from build123d import *

# Parameters (mm, degrees)
ESBO_O1_W                     = 13
ESBO_O1_H                     = 15
RESSALTO_EXTRUS_O1_DEPTH      = 9.5
ESBO_O3_R                     = 6.25
CORTE_EXTRUS_O1_DEPTH         = 10.5
ESBO_O2_W                     = 3
ESBO_O2_H                     = 4
ESBO_O2_R                     = 0.75
RESSALTO_EXTRUS_O2_DEPTH      = 8
RESSALTO_EXTRUS_O2_DEPTH_BACK = 9.5
RESSALTO_EXTRUS_O3_DEPTH      = 1.5
ESBO_O5_W                     = 12
ESBO_O5_H                     = 10
ESBO_O5_W_2                   = 10
ESBO_O5_H_2                   = 8
RESSALTO_EXTRUS_O4_DEPTH      = 7.5
RESSALTO_EXTRUS_O5_DEPTH      = 1
FILETE1_R                     = 1


with BuildPart() as part:
    # Esbo_o1 → Ressalto-extrus_o1 (new body)
    with BuildSketch(Plane.XY):
        Rectangle(ESBO_O1_W, ESBO_O1_H)
    extrude(amount=-RESSALTO_EXTRUS_O1_DEPTH)

    # Esbo_o3 → Corte-extrus_o1 (cut, through all)
    with BuildSketch(Plane.XY):
        Circle(ESBO_O3_R)
    extrude(amount=-CORTE_EXTRUS_O1_DEPTH, mode=Mode.SUBTRACT)

    # Esbo_o4 → Ressalto-extrus_o3 (add)
    with BuildSketch(Plane.ZY.offset(6.5)):
        Polygon((-6.5, 2.25), (-6.5, -1.75), (-4.849272887, -0.75), (-4.849272887, 1.25), align=None)
    extrude(amount=RESSALTO_EXTRUS_O3_DEPTH)

    # Esbo_o5 → Ressalto-extrus_o4 (add)
    with BuildSketch(Plane(origin=(0, 0, -9.5), x_dir=(-1, 0, 0), z_dir=(0, 0, -1))):
        Rectangle(ESBO_O5_W, ESBO_O5_H)
        Rectangle(ESBO_O5_W_2, ESBO_O5_H_2, mode=Mode.SUBTRACT)
    extrude(amount=-RESSALTO_EXTRUS_O4_DEPTH)



with BuildPart() as body_2:
    # Esbo_o2 → Ressalto-extrus_o2 (new body, two sides)
    with BuildSketch(Plane.XY) as ressalto_extrus_o2_sk:
        Rectangle(ESBO_O2_W, ESBO_O2_H)
        Circle(ESBO_O2_R, mode=Mode.SUBTRACT)
    extrude(amount=RESSALTO_EXTRUS_O2_DEPTH)
    extrude(ressalto_extrus_o2_sk.sketch, amount=-RESSALTO_EXTRUS_O2_DEPTH_BACK)


with BuildPart() as part_1:
    add(part.part)

    add(body_2.part)  # Ressalto-extrus_o5 merges body 2
    # Esbo_o6 → Ressalto-extrus_o5 (add)
    with BuildSketch(Plane.ZY.offset(1.5)):
        Polygon((-1, 7.5), (-1, 6.5), (2, 3.667217521), (2, -3.332782479), (-1, -6.5), (-1, -7.5), (-2, -7.5), (-2, -6.101577834), (1, -2.934360312), (1, 3.236113484), (-2, 6.068895963), (-2, 7.5), align=None)
    ressalto_extrus_o5 = extrude(amount=RESSALTO_EXTRUS_O5_DEPTH)

    # Espelhar1: Ressalto-extrus_o5 across plane
    add(ressalto_extrus_o5.mirror(Plane(origin=(0, 0, 0), x_dir=(0, 0, 1), z_dir=(1, 0, 0))))

    # Filete1
    filete1_edges = [part_1.edges().sort_by_distance(p)[0] for p in [
        (2, -3.332782479, 2),
        (2, 3.667217521, 2),
        (-2, -3.332782479, 2),
        (-2, 3.667217521, 2),
    ]]
    fillet(filete1_edges, radius=FILETE1_R)


solid = part_1.part
The listing builds one solid part. Answer for the finished solid, in the listing's coordinates (mm). A direction names the side the tool comes from. Round coordinates to 2 decimals unless told otherwise and drop trailing zeros. Write each loop counter-clockwise with the first axis right and the second up, starting at its lowest first coordinate (ties: lowest second). Pieces come first, ordered by that corner, then holes. Notation, with made-up numbers: (73.25, -2) - (77.25, -2) arc R31 ccw to (77.25, 22) - close; hole circle Ø2 at (-31, -39.75). An arc over 180 degrees is marked (long way). Use a Markdown table: item, result. Add a question column.
1. The part is cut by section D-D (z = 6.5). Write down the section's boundary in (x, y), and give its area (3 significant figures).
2. The part is cut by section A-A (x = 0). Write down the section's boundary in (y, z), and give its area (3 significant figures).
3. The part is cut by section C-C (y = -1.5). Give the number of separate pieces and of enclosed holes in the cut face, and give its area (3 significant figures).
4. Consider line 1 (Y direction, x = 0, z = -5); line 2 (Y direction, x = 1.75, z = -7); line 3 (X direction, y = 1, z = -5.5). Determine where each line is inside the solid, lowest interval first.
5. The part is cut by section B-B (z = -7). Write down the section's boundary in (x, y).
6. A tool of negligible diameter and unlimited length cuts with its end or side. For faces 4 (the face through (-1.5, 0, 5)), 5 (the face through (1.5, 0, -4)), 6 (the face through (5, 0, -6)), 7 (the face through (-1.993, 5.03, 0.557)), 8 (the face through (-1.99, -4.52, -0.5)), from which of +Z, -Z, +X, -X, +Y, -Y can it reach the whole face along a straight path? Write none if from no direction.
7. Flat-ended cylindrical pins translate along their axes: P1, Ø5, axis at x = -1, z = 3.5, coming from the +Y side; P2, Ø1, axis at y = -1, z = 4, coming from the -X side; P3, Ø0.8, axis at x = -5.5, y = -1.5, coming from the +Z side. Find the tip coordinate at first contact, or state that the pin passes through.
8. For a pull along Y with two mould halves and no side action, classify faces 1 (the face through (6.5, 0, -5)), 2 (the face through (-7.24, -1.26, -5.69)), 3 (the face through (0, 5, -6)) as +Y half, -Y half, draft (parallel to the pull), parting line (faces both ways), or undercut.
Reported:
| question | item | result |
|---|---|---|
| 1 | outline | (-1.5, -2) - (1.5, -2) - (1.5, 2) - (-1.5, 2) - close; hole circle Ø1.5 at (0, 0) |
| 1 | area | 10.2 mm^2 |
| 2 | outline | (-7.5, -9.5) - (-6.25, -9.5) - (-6.25, 0) - (-7.5, 0) - close; (-5, -9.5) - (-4, -9.5) - (-4, -2) - (-5, -2) - close; (-2, -9.5) - (-0.75, -9.5) - (-0.75, 8) - (-2, 8) - close; (0.75, -9.5) - (2, -9.5) - (2, 8) - (0.75, 8) - close; (4, -9.5) - (5, -9.5) - (5, -2) - (4, -2) - close; (6.25, -9.5) - (7.5, -9.5) - (7.5, 0) - (6.25, 0) - close |
| 2 | area | 82.5 mm^2 |
| 3 | separate pieces | 5 |
| 3 | enclosed holes | 0 |
| 3 | area | 78.3 mm^2 |
| 4 | line 1 | -7.5 to -6.25, -5 to -4, -2 to -0.75, 0.75 to 2, 4 to 5, 6.25 to 7.5 |
| 4 | line 2 | -7.5 to -6, -5 to -4, 4 to 5, 6 to 7.5 |
| 4 | line 3 | -8 to -6.17, -6 to -5, -1.5 to 1.5, 5 to 6, 6.17 to 6.5 |
| 5 | outline | (-6.5, -7.5) - (6.5, -7.5) - (6.5, 7.5) - (-6.5, 7.5) - close; (-1.5, -2) - (1.5, -2) - (1.5, 2) - (-1.5, 2) - close; hole (-6, -1.75) - (-6, 1.75) arc R6.25 ccw to start; hole (-5, -3.75) arc R6.25 ccw to (-4.8, -4) - (4.8, -4) arc R6.25 ccw to (5, -3.75) - (5, 3.75) arc R6.25 ccw to (4.8, 4) - (-4.8, 4) arc R6.25 ccw to (-5, 3.75) - close; hole (-3.75, -5) arc R6.25 ccw to (3.75, -5) - close; hole (-3.75, 5) - (3.75, 5) arc R6.25 ccw to start; hole circle Ø1.5 at (0, 0); hole (6, -1.75) arc R6.25 ccw to (6, 1.75) - close |
| 6 | face 4 | +Z, -X, +Y, -Y |
| 6 | face 5 | -Z |
| 6 | face 6 | +Z, -Z |
| 6 | face 7 | +Z |
| 6 | face 8 | none |
| 7 | P1 | y = 4.56 |
| 7 | P2 | x = -1.5 |
| 7 | P3 | z = -2 |
| 8 | face 1 | draft |
| 8 | face 2 | -Y half |
| 8 | face 3 | undercut |
